Can you work these out from the model? Positions are in its coordinate system, mm. A direction names the side the tool comes from. Round coordinates to 2 decimals unless told otherwise and drop trailing zeros. Write each loop counter-clockwise with the first axis right and the second up, starting at its lowest first coordinate (ties: lowest second). Pieces come first, ordered by that corner, then holes. Notation, with made-up numbers: M -25,-14 L -8,-14 A10 ccw -8,-3 Z; hole C 57.5,81.25 d8. An arc over 180 degrees is marked long. Answer in a Markdown table with one row per item. Add a question column.
(1) For faces 4 (the face through (62.643, 4.042, -0.872)), 5 (the face through (-35, 3, 7)), 6 (the face through (-61.453, 0.493, 0.716)), 7 (the face through (15.466, 3.451, -8.184)), 8 (the face through (-1, 7, 12)), which set-ups out of +Z, -Z, +X, -X, +Y, -Y let a thin tool reach every point of the face, with its end or its side?
(2) I'm going to push flat-ended pins straight in: pin 1 (1 mm diameter, centred on x = -49.5, y = 5, fed in from +Z); pin 2 (12 mm diameter, centred on x = -56, z = 0, fed in from +Y); pin 3 (1 mm diameter, centred on x = -20, y = 4, fed in from +Z). Where does each tip first touch, or does it pass through?
(3) Suppose I cut it at A-A, the plane x = 56. Write out the boundary of the cut face in (y, z).
(4) If I drill on probe 1 along Z at (x, y) = (56, 0.7); probe 2 along X at (y, z) = (2.75, -2); probe 3 along X at (y, z) = (4.25, 1), over which ranges is the centre line in solid material (lowest first)?
(5) If we mould it in two halves opening along Z, with no side actions, what happens to faces 1 (the face through (-15.466, 3.451, 8.184)), 2 (the face through (59, 1, -5)), 3 (the face through (-15.24, 3.45, -8.25))? For each: released by +Z, released by -Z, zero draft, split by the parting line, or undercut.
(6) Suppose I cut it at C-C, the plane x = 0. Write out the boundary of the cut face in (y, z).
(7) Suppose I cut it at B-B, the plane y = 4. Write out the boundary of the cut face in (x, z).
(8) Suppose I cut it at D-D, the plane x = -25. Write out the boundary of the cut face in (y, z).
from build123d import *

# Parameters (mm, degrees)
SKETCH_1_R          = 10
SKETCH_1_R_2        = 5.5
SKETCH_1_R_3        = 1.6
EXTRUDE_1_DEPTH     = 7
SKETCH_3_R          = 6.55
SKETCH_3_R_2        = 6.7
CUT_EXTRUDE_1_DEPTH = 6
SKETCH_4_R          = 11.3
CUT_EXTRUDE_2_DEPTH = 6


with BuildPart() as part:
    # Эскиз1 → Бобышка-Вытянуть1 (new body)
    with BuildSketch(Plane(origin=(0, 0, 0), x_dir=(1, 0, 0), z_dir=(0, 1, 0))):
        with BuildLine():
            Line((-23.8117618, 7), (-45.464346247, 7))
            ThreePointArc((-45.464346247, 7), (-48.202959035, 7.382307969), (-50.732173124, 8.5))
            ThreePointArc((-50.732173124, 8.5), (-66, 0), (-50.732173124, -8.5))
            ThreePointArc((-50.732173124, -8.5), (-48.202959035, -7.382307969), (-45.464346247, -7))
            Line((-45.464346247, -7), (-23.8117618, -7))
            ThreePointArc((-23.8117618, -7), (-15.350620677, -8.217903292), (-7.576469664, -11.772727273))
            ThreePointArc((-7.576469664, -11.772727273), (0, -14), (7.576469664, -11.772727273))
            ThreePointArc((7.576469664, -11.772727273), (15.350620677, -8.217903292), (23.8117618, -7))
            Line((23.8117618, -7), (45.464346247, -7))
            ThreePointArc((45.464346247, -7), (48.202959035, -7.382307969), (50.732173124, -8.5))
            ThreePointArc((50.732173124, -8.5), (66, 0), (50.732173124, 8.5))
            ThreePointArc((50.732173124, 8.5), (48.202959035, 7.382307969), (45.464346247, 7))
            Line((45.464346247, 7), (23.8117618, 7))
            ThreePointArc((23.8117618, 7), (15.350620677, 8.217903292), (7.576469664, 11.772727273))
            ThreePointArc((7.576469664, 11.772727273), (0, 14), (-7.576469664, 11.772727273))
            ThreePointArc((-7.576469664, 11.772727273), (-15.350620677, 8.217903292), (-23.8117618, 7))
        make_face()
        with Locations(Location((0, 0, 0), (0, 0, 270))):
            Circle(SKETCH_1_R, mode=Mode.SUBTRACT)
        with Locations(Location((56, 0, 0), (0, 0, 270))):
            Circle(SKETCH_1_R_2, mode=Mode.SUBTRACT)
        with Locations(Location((-56, 0, 0), (0, 0, 90))):
            Circle(SKETCH_1_R_2, mode=Mode.SUBTRACT)
        with Locations(Location((-30, 0, 0), (0, 0, 270))):
            Circle(SKETCH_1_R_3, mode=Mode.SUBTRACT)
        with Locations(Location((30, 0, 0), (0, 0, 270))):
            Circle(SKETCH_1_R_3, mode=Mode.SUBTRACT)
    extrude(amount=EXTRUDE_1_DEPTH)

    # Эскиз3 → Вырез-Вытянуть1 (cut)
    with BuildSketch(Plane(origin=(0, 7, 0), x_dir=(1, 0, 0), z_dir=(0, 1, 0))):
        with Locations(Location((-56, 0, 0), (0, 0, 270))):
            Circle(SKETCH_3_R)
        with Locations(Location((56, 0, 0), (0, 0, 270))):
            Circle(SKETCH_3_R_2)
    extrude(amount=-CUT_EXTRUDE_1_DEPTH, mode=Mode.SUBTRACT)

    # Эскиз4 → Вырез-Вытянуть2 (cut)
    with BuildSketch(Plane(origin=(0, 7, 0), x_dir=(1, 0, 0), z_dir=(0, 1, 0))):
        with Locations(Location((0, 0, 0), (0, 0, 270))):
            Circle(SKETCH_4_R)
    extrude(amount=-CUT_EXTRUDE_2_DEPTH, mode=Mode.SUBTRACT)


solid = part.part
Calculated:
| question | item | result |
|---|---|---|
| 1 | face 4 | +Y |
| 1 | face 5 | +Z, +Y, -Y |
| 1 | face 6 | +Y, -Y |
| 1 | face 7 | -Z, +Y, -Y |
| 1 | face 8 | +Z, -Z, +X, -X, +Y |
| 2 | pin 1 | z = 8.09 |
| 2 | pin 2 | y = 1 |
| 2 | pin 3 | z = 7.31 |
| 3 | outline | M 0,-10 L 7,-10 L 7,-6.7 L 1,-6.7 L 1,-5.5 L 0,-5.5 Z; M 0,5.5 L 1,5.5 L 1,6.7 L 7,6.7 L 7,10 L 0,10 Z |
| 4 | probe 1 | -10 to -5.5, 5.5 to 10 |
| 4 | probe 2 | -65.8 to -62.24, -49.76 to -11.12, 11.12 to 49.61, 62.39 to 65.8 |
| 4 | probe 3 | -65.95 to -62.47, -49.53 to -31.25, -28.75 to -11.26, 11.26 to 28.75, 31.25 to 49.38, 62.62 to 65.95 |
| 5 | face 1 | released by +Z |
| 5 | face 2 | undercut |
| 5 | face 3 | released by -Z |
| 6 | outline | M 0,-14 L 7,-14 L 7,-11.3 L 1,-11.3 L 1,-10 L 0,-10 Z; M 0,10 L 1,10 L 1,11.3 L 7,11.3 L 7,14 L 0,14 Z |
| 7 | outline | M -50.73,-8.5 A10 cw -45.46,-7 L -23.81,-7 A30 cw -7.58,-11.77 A14 ccw 7.58,-11.77 A30 cw 23.81,-7 L 45.46,-7 A10 cw 50.73,-8.5 A10 ccw long 50.73,8.5 A10 cw 45.46,7 L 23.81,7 A30 cw 7.58,11.77 A14 ccw -7.58,11.77 A30 cw -23.81,7 L -45.46,7 A10 cw -50.73,8.5 A10 ccw long Z; hole C -56,0 d13.1; hole C -30,0 d3.2; hole C 0,0 d22.6; hole C 30,0 d3.2; hole C 56,0 d13.4 |
| 8 | outline | M 0,-7 L 7,-7 L 7,7 L 0,7 Z |
